```python
from build123d import *

# Parameters (mm, degrees)
F0_W     = 63.5
F0_H     = 63.5
F1_DEPTH = 25.4
F2_W     = 48.26
F2_H     = 48.26
F3_DEPTH = 17.78
F4_W     = 48.26
F4_H     = 7.62
F5_DEPTH = 5.08
F6_W     = 1.774852
F6_H     = 2.54
F7_DEPTH = 58.42


with BuildPart() as f1:
    # F0 (on Top) → F1 (new body)
    with BuildSketch(Plane.XY):
        with Locations((-13.989703, 19.433425)):
            Rectangle(F0_W, F0_H)
    extrude(amount=F1_DEPTH)

    # F2 (on face) → F3 (cut)
    with BuildSketch(Plane.XY.offset(25.4)):
        with Locations((-13.989703, 19.433425)):
            Rectangle(F2_W, F2_H)
    extrude(amount=-F3_DEPTH, mode=Mode.SUBTRACT)

    # F4 (on face) → F5 (cut)
    with BuildSketch(Plane.XY.offset(25.4)):
        with Locations((-13.989703, -8.506575)):
            Rectangle(F4_W, F4_H)
    extrude(amount=-F5_DEPTH, mode=Mode.SUBTRACT)

    # F6 (on face) → F7 (cut)
    with BuildSketch(Plane.XZ.offset(12.316575)):
        with Locations((-39.007129, 21.59)):
            Rectangle(F6_W, F6_H)
    extrude(amount=-F7_DEPTH, mode=Mode.SUBTRACT)


solid = f1.part
```
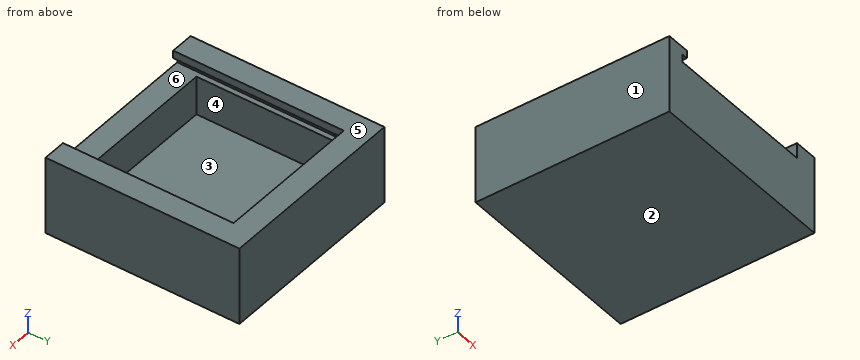
Check sheet for the modelled part. Datum: model origin and axes. Units: mm. Face numbers are marked on the shaded views. A direction names the side the tool comes from. Give positions to 0.01 mm unless a question says otherwise; leave off trailing zeros. Write each loop counter-clockwise with the first axis right and the second up, starting at its lowest first coordinate (ties: lowest second). Pieces come first, ordered by that corner, then holes. Notation, with made-up numbers: (-40, 76.5) - (-4, 76.5) arc R17 ccw to (-4, 85.5) - close; hole circle Ø6 at (70, 84). An arc over 180 degrees is marked (long way). Answer as a JSON object with one key per item and string values. Group by question number.
1) Sectioned sample at A-A (z = 23.75). Record the cut outline in (x, y).
2) Sectioned sample at C-C (x = 7.5). Record the cut outline in (y, z).
3) Sectioned sample at D-D (z = 19). Record the cut outline in (x, y), then the cut area to 3 significant figures.
4) Access from +Z, -Z, +X, -X, +Y, -Y to the whole of each face (thin tool, end or side, straight path). Record for the marked faces 4, 5 and 6.
5) Thickness scan on probe 1 along X at (y, z) = (24, 8.25); probe 2 along Y at (x, z) = (-32, 16.5); probe 3 along Z at (x, y) = (-7, 35). Record the ranges inside material, lowest first. Write a range as from..to.
6) Depth check by flat-ended pin: P1, Ø4, axis at x = 7, y = -5.5, coming from the -Z side; P2, Ø1.5, axis at x = -24.5, y = 37.5, coming from the +Z side; P3, Ø0.5, axis at x = -39, z = 21, coming from the -Y side. Enter the tip coordinate at first touch or a pass-through.
7) Release check for a two-part mould opening along X. For the marked faces 1, 2 and 3 record: pulls with the +X half, pulls with the -X half, needs draft (parallel to the pull), parting line crosses it, or undercut.
8) Sectioned sample at B-B (y = 17). Record the cut outline in (x, z), then the cut area to 3 significant figures.
Geometry results:
{
 "1": {"outline": "(-45.74, -12.32) - (-38.12, -12.32) - (-38.12, 43.56) - (10.14, 43.56) - (10.14, -12.32) - (17.76, -12.32) - (17.76, 51.18) - (-45.74, 51.18) - close"},
 "2": {"outline": "(-12.32, 0) - (51.18, 0) - (51.18, 25.4) - (43.56, 25.4) - (43.56, 7.62) - (-4.7, 7.62) - (-4.7, 20.32) - (-12.32, 20.32) - close"},
 "3": {"outline": "(-45.74, -12.32) - (17.76, -12.32) - (17.76, 51.18) - (-45.74, 51.18) - close; hole (-38.12, -4.7) - (10.14, -4.7) - (10.14, 43.56) - (-38.12, 43.56) - close", "area": "1,700 mm^2"},
 "4": {"face 4": "+Z", "face 5": "+Z, +X, -X, +Y, -Y", "face 6": "-Y"},
 "5": {"probe 1": "x = -45.74..-38.12, 10.14..17.76", "probe 2": "y = -12.32..-4.7, 43.56..51.18", "probe 3": "z = 0..7.62"},
 "6": {"P1": "stops at z = 0", "P2": "stops at z = 7.62", "P3": "stops at y = 46.1"},
 "7": {"face 1": "pulls with the -X half", "face 2": "needs draft", "face 3": "undercut"},
 "8": {"outline": "(-45.74, 0) - (17.76, 0) - (17.76, 25.4) - (10.14, 25.4) - (10.14, 7.62) - (-38.12, 7.62) - (-38.12, 20.32) - (-39.89, 20.32) - (-39.89, 22.86) - (-38.12, 22.86) - (-38.12, 25.4) - (-45.74, 25.4) - close", "area": "750 mm^2"}
}
